Check sheet for the modelled part. Datum: model origin and axes. Units: mm. Face numbers are marked on the shaded views. A direction names the side the tool comes from. Give positions to 0.01 mm unless a question says otherwise; leave off trailing zeros. Loops run counter-clockwise (first coordinate to the right, second up) from the corner with the lowest first, then second, coordinate; pieces in that order, holes last. Notation, with made-up numbers: M 64,7.5 L 69,7.5 A12 ccw 69,26.5 Z; hole C -19.5,13 d8. An arc over 180 degrees is marked long. Use one line per item in the form item = value.
Solid Edge part; units mm, degrees
sketch "Sketch1" plane through (0, 0, 0) normal (0, -1, 0) x (1, 0, 0)
  line L0 (4.6188, 8) -> (-4.6188, 8)
  line L1 (-4.6188, 8) -> (-9.2376, 0)
  line L2 (-9.2376, 0) -> (-4.6188, -8)
  line L3 (-4.6188, -8) -> (4.6188, -8)
  line L4 (4.6188, -8) -> (9.2376, 0)
  line L5 (9.2376, 0) -> (4.6188, 8)
  circle A0 centre (0, 0) radius 5
extrude "Protrusion1" add sketch "Sketch1" along normal mid plane 8.04
sketch "Sketch2" plane through (0, 0, 0) normal (0, 0, 1) x (1, 0, 0)
  line L0 (-9.2376, 3.215) -> (-19.2376, 3.215)
  line L1 (-19.2376, 3.215) -> (-19.2376, 14.02)
  line L2 (-19.2376, 14.02) -> (-8, 14.02)
  line L3 (-8, 14.02) -> (-8, 4.02)
  line L4 (-8, 4.02) -> (-9.2376, 3.215)
revolve "RevolvedCutout1" cut sketch "Sketch2" angle 360 about axis through (0, 0, 0) along (0, 1, 0)
mirror "Mirror1" about plane through (0, 0, 0) normal (0, -1, 0) of "RevolvedCutout1"
sketch "Sketch3" plane through (0, -4.02, 0) normal (0, -1, 0) x (1, 0, 0)
  circle A0 centre (0, 0) radius 8
  circle A1 centre (0, 0) radius 5
extrude "Protrusion2" add sketch "Sketch3" along normal blind 3.86
fillet "Round1" radius 1 1 edges at (-8, -7.88, 0)
cosmetic_thread "Thread1"
properties material "Stainless steel"
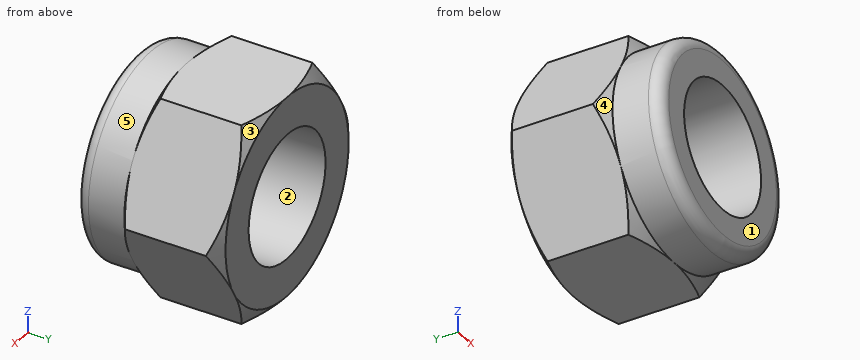
1) Section check A-A (y = -2.75). Record the cut outline in (x, z).
Evaluation:
outline = M -9.24,0 L -4.62,-8 L 4.62,-8 L 9.24,0 L 4.62,8 L -4.62,8 Z; hole C 0,0 d10
2) Set-up check for the marked faces 4 and 5: record each of +Z, -Z, +X, -X, +Y, -Y from which the full face is reachable in a straight line by a thin tool's end or side.
Evaluation:
face_4 = -X, -Y
face_5 = -Y
3) Release check for a two-part mould opening along Z. For the marked faces 1, 2 and 3 record: pulls with the +Z half, pulls with the -Z half, needs draft (parallel to the pull), parting line crosses it, or undercut.
Evaluation:
face_1 = needs draft
face_2 = undercut
face_3 = pulls with the +Z half
4) Section check B-B (y = -6). Record the cut outline in (x, z).
Evaluation:
outline = C 0,0 d16; hole C 0,0 d10
5) Scan lines: line 1 (Z direction, x = 0, y = -3.75); line 2 (X direction, y = -4.25, z = 3.5); line 3 (X direction, y = 3.75, z = 2.25). Record each from-to range of solid material in increasing order.
Evaluation:
line_1 = -8 to -5, 5 to 8
line_2 = -7.19 to -3.57, 3.57 to 7.19
line_3 = -7.94 to -4.47, 4.47 to 7.94
6) Depth check by flat-ended pin: pin 1 Ø2 at (y, z) = (0.5, -5.5) entering from -X; pin 2 Ø1 at (x, y) = (-7.5, -1) entering from +Z; pin 3 Ø4 at (x, y) = (7, -5.5) entering from +Z (3 decimals). Enter the tip coordinate at first touch or a pass-through.
Evaluation:
pin_1 = -6.64
pin_2 = 3.88
pin_3 = 6.245
